from build123d import *

# Parameters (mm, degrees)
CROQUIS18_W                  = 39
CROQUIS18_H                  = 54
SALIENTE_EXTRUIR8_DEPTH      = 40.280661595
SALIENTE_EXTRUIR9_REACH      = 87.298
SALIENTE_EXTRUIR9_END_RADIUS = 16
SALIENTE_EXTRUIR10_DEPTH     = 26.5
CORTAR_EXTRUIR8_START        = -39
CROQUIS22_R                  = 15
CORTAR_EXTRUIR8_DEPTH        = 39
CORTAR_EXTRUIR9_DEPTH        = 84.025081472
CROQUIS24_W                  = 10.8
CROQUIS24_H                  = 54
CORTAR_EXTRUIR10_DEPTH       = 12
CROQUIS25_R                  = 2.25
CORTAR_EXTRUIR11_DEPTH       = 24.2
REDONDEO1_R                  = 2
REDONDEO2_R                  = 2
CROQUIS26_R                  = 2.25
CORTAR_EXTRUIR12_DEPTH       = 30
CROQUIS27_W                  = 15
CROQUIS27_H                  = 15
CORTAR_EXTRUIR13_DEPTH       = 101.562974791


with BuildPart() as part:
    # Croquis18 → Saliente-Extruir8 (new body)
    with BuildSketch(Plane(origin=(0, 0, 0), x_dir=(1, 0, 0), z_dir=(0, 1, 0))):
        with Locations((49.353088131, -3.207737261)):
            Rectangle(CROQUIS18_W, CROQUIS18_H)
    extrude(amount=SALIENTE_EXTRUIR8_DEPTH)

    # Saliente-Extruir9: up to this cylinder (the profile starts outside it)
    saliente_extruir9_end = Plane(origin=(39.1607, 58.280661595, 3.207737261), z_dir=(1, 0, 0)) * Cylinder(SALIENTE_EXTRUIR9_END_RADIUS, 207.596, mode=Mode.PRIVATE)
    # Croquis20 → Saliente-Extruir9 (add, up to the surface)
    with BuildSketch(Plane(origin=(0, 40.280661595, 0), x_dir=(1, 0, 0), z_dir=(0, 1, 0)), mode=Mode.PRIVATE) as saliente_extruir9_sk1:
        Polygon((38.853088131, -11.507737261), (38.853088131, -14.207737261), (60.353088131, -14.207737261), (60.353088131, 7.792262739), (38.853088131, 7.792262739), (38.853088131, 5.092262739), (56.853088131, 5.092262739), (56.853088131, -11.507737261), align=None)
    saliente_extruir9_tool1 = extrude(saliente_extruir9_sk1.sketch, amount=SALIENTE_EXTRUIR9_REACH, mode=Mode.PRIVATE) - saliente_extruir9_end
    add(saliente_extruir9_tool1.solids().sort_by_distance((39.1607, 40.280662, 12.857737))[0])

    # Croquis21 → Saliente-Extruir10 (add)
    with BuildSketch(Plane(origin=(0, 40.280661595, 0), x_dir=(1, 0, 0), z_dir=(0, 1, 0))):
        Polygon((68.853088131, 23.792262739), (29.853088131, 23.792262739), (29.853088131, 7.792262739), (60.353088131, 7.792262739), (60.353088131, -14.207737261), (29.853088131, -14.207737261), (29.853088131, -30.207737261), (68.853088131, -30.207737261), align=None)
    extrude(amount=SALIENTE_EXTRUIR10_DEPTH)

    # Croquis22 → Cortar-Extruir8 (cut)
    with BuildSketch(Plane(origin=(68.853088131, 0, 0), x_dir=(0, 0, -1), z_dir=(1, 0, 0)).offset(CORTAR_EXTRUIR8_START)):
        with Locations((-3.207737261, 58.280661595)):
            Circle(CROQUIS22_R)
    extrude(amount=CORTAR_EXTRUIR8_DEPTH, mode=Mode.SUBTRACT)

    # Croquis23 → Cortar-Extruir9 (cut, through all)
    with BuildSketch(Plane(origin=(68.853088131, 0, 0), x_dir=(0, 0, -1), z_dir=(1, 0, 0))):
        with BuildLine():
            Line((-15.566944355, 66.780661595), (-18.207737261, 66.780661595))
            Line((-18.207737261, 66.780661595), (-18.207737261, 58.280661595))
            ThreePointArc((-18.207737261, 58.280661595), (-17.532333353, 62.731048859), (-15.566944355, 66.780661595))
        make_face()
        with BuildLine():
            ThreePointArc((9.151469833, 66.780661595), (11.116858831, 62.731048859), (11.792262739, 58.280661595))
            Line((11.792262739, 58.280661595), (11.792262739, 66.780661595))
            Line((11.792262739, 66.780661595), (9.151469833, 66.780661595))
        make_face()
    extrude(amount=-CORTAR_EXTRUIR9_DEPTH, mode=Mode.SUBTRACT)

    # Croquis24 → Cortar-Extruir10 (cut)
    with BuildSketch(Plane(origin=(0, 66.780661595, 0), x_dir=(1, 0, 0), z_dir=(0, 1, 0))):
        with Locations((35.253088131, -3.207737261)):
            Rectangle(CROQUIS24_W, CROQUIS24_H)
    extrude(amount=-CORTAR_EXTRUIR10_DEPTH, mode=Mode.SUBTRACT)

    # Croquis25 → Cortar-Extruir11 (cut)
    with BuildSketch(Plane.ZY.offset(-40.653088131)):
        with Locations(Location((20.707737261, 58.280661595, 0), (0, 0, 270))):
            Circle(CROQUIS25_R)
        with Locations(Location((-14.292262739, 58.280661595, 0), (0, 0, 270))):
            Circle(CROQUIS25_R)
    extrude(amount=-CORTAR_EXTRUIR11_DEPTH, mode=Mode.SUBTRACT)

    # Redondeo1
    redondeo1_edges = [part.edges().sort_by_distance(p)[0] for p in [
        (68.853088131, 62.530661595, 18.207737261),
        (68.853088131, 62.530661595, -11.792262739),
        (68.853088131, 33.390330798, -23.792262739),
        (54.753088131, 66.780661595, 30.207737261),
        (29.853088131, 27.390330798, 30.207737261),
        (68.853088131, 33.390330798, 30.207737261),
        (29.853088131, 27.390330798, -23.792262739),
        (29.853088131, 51.200842989, -10.016338076),
        (29.853088131, 54.780661595, -17.585238812),
        (29.853088131, 54.780661595, 24.000713334),
        (40.653088131, 60.780661595, -23.792262739),
        (35.253088131, 54.780661595, -23.792262739),
        (35.253088131, 54.780661595, 30.207737261),
        (40.653088131, 60.780661595, 30.207737261),
        (29.853088131, 40.280661595, 3.207737261),
        (49.353088131, 0, -23.792262739),
        (68.853088131, 0, 3.207737261),
        (68.853088131, 66.780661595, 24.207737261),
        (54.753088131, 66.780661595, -23.792262739),
        (49.353088131, 0, 30.207737261),
        (29.853088131, 0, 3.207737261),
        (29.853088131, 44.181642082, -7.792262739),
        (29.853088131, 44.181642082, 14.207737261),
        (29.853088131, 51.200842989, 16.431812597),
        (68.853088131, 43.280661596, 3.207737261),
        (68.853088131, 66.780661595, -17.792262739),
    ]]
    fillet(redondeo1_edges, radius=REDONDEO1_R)

    # Redondeo2
    # the kernel refuses this fillet: 2 mm, written as the material it takes off along each edge
    with BuildSketch(Plane(origin=(66.853088131, 64.780661595, -13.792262739), x_dir=(0, 1, 0), z_dir=(0, 0, 1))) as redondeo2_piece_1_section:
        Polygon((0, 0), (REDONDEO2_R, 0), (REDONDEO2_R, -REDONDEO2_R), (0, -REDONDEO2_R), align=None)
    redondeo2_piece_1 = extrude(amount=REDONDEO2_R, mode=Mode.PRIVATE)
    redondeo2_piece_1 = redondeo2_piece_1 - Plane(origin=(66.853088131, 64.780661595, -13.792262739), x_dir=(-0.7071067811865475, -0.7071067811865476, 0), z_dir=(0, 0, 1)) * Sphere(REDONDEO2_R, mode=Mode.PRIVATE)
    add(redondeo2_piece_1, mode=Mode.SUBTRACT)
    with BuildSketch(Plane(origin=(66.853088131, 64.780661595, 20.207737261), x_dir=(0, 0, -1), z_dir=(0, 1, 0))) as redondeo2_piece_2_section:
        Polygon((0, 0), (REDONDEO2_R, 0), (REDONDEO2_R, -REDONDEO2_R), (0, -REDONDEO2_R), align=None)
    redondeo2_piece_2 = extrude(amount=REDONDEO2_R, mode=Mode.PRIVATE)
    redondeo2_piece_2 = redondeo2_piece_2 - Plane(origin=(66.853088131, 64.780661595, 20.207737261), x_dir=(-0.7071067811865475, 0, 0.7071067811865475), z_dir=(0, 1, 0)) * Sphere(REDONDEO2_R, mode=Mode.PRIVATE)
    add(redondeo2_piece_2, mode=Mode.SUBTRACT)
    with BuildSketch(Plane(origin=(42.653088131, 64.780661595, -21.792262739), x_dir=(0, 1, 0), z_dir=(-1, 0, 0))) as redondeo2_piece_3_section:
        Polygon((0, 0), (REDONDEO2_R, 0), (REDONDEO2_R, REDONDEO2_R), (0, REDONDEO2_R), align=None)
    redondeo2_piece_3 = extrude(amount=REDONDEO2_R, mode=Mode.PRIVATE)
    redondeo2_piece_3 = redondeo2_piece_3 - Plane(origin=(42.653088131, 64.780661595, -21.792262739), x_dir=(0, -0.7071067811865475, 0.7071067811865475), z_dir=(-1, 0, 0)) * Sphere(REDONDEO2_R, mode=Mode.PRIVATE)
    add(redondeo2_piece_3, mode=Mode.SUBTRACT)
    with BuildSketch(Plane(origin=(42.653088131, 64.780661595, 28.207737261), x_dir=(-1, 0, 0), z_dir=(0, 1, 0))) as redondeo2_piece_4_section:
        Polygon((0, 0), (REDONDEO2_R, 0), (REDONDEO2_R, REDONDEO2_R), (0, REDONDEO2_R), align=None)
    redondeo2_piece_4 = extrude(amount=REDONDEO2_R, mode=Mode.PRIVATE)
    redondeo2_piece_4 = redondeo2_piece_4 - Plane(origin=(42.653088131, 64.780661595, 28.207737261), x_dir=(0.7071067811865475, 0, -0.7071067811865476), z_dir=(0, 1, 0)) * Sphere(REDONDEO2_R, mode=Mode.PRIVATE)
    add(redondeo2_piece_4, mode=Mode.SUBTRACT)
    with BuildSketch(Plane(origin=(66.853088131, 66.780661595, 18.207737261), x_dir=(0, -1.5546675058430992e-10, 1.0), z_dir=(-1, 0, 0)), Plane(origin=(66.853088131, 66.780661595, -11.792262739), x_dir=(0, -1, 0), z_dir=(-1, 0, 0))) as redondeo2_piece_5:
        with BuildLine():
            CenterArc((REDONDEO2_R, -REDONDEO2_R), REDONDEO2_R, 90.000000009, 90)
            Line((REDONDEO2_R * 1.55466750608e-10, -REDONDEO2_R), (0, 0))
            Line((0, 0), (REDONDEO2_R, 0))
        make_face()
    extrude(amount=31.200000001, mode=Mode.SUBTRACT)
    with BuildSketch(Plane(origin=(40.653088131, 66.780661595, -6.792262738), x_dir=(0, -1, 0), z_dir=(0, 0, -1))) as redondeo2_piece_6:
        with BuildLine():
            CenterArc((REDONDEO2_R, -REDONDEO2_R), REDONDEO2_R, 90, 90)
            Line((0, -REDONDEO2_R), (0, 0))
            Line((0, 0), (REDONDEO2_R, 0))
        make_face()
    extrude(amount=15.000000001, mode=Mode.SUBTRACT)
    with BuildSketch(Plane(origin=(40.653088131, 66.780661595, 28.207737261), x_dir=(1.0, -1.5546675058430992e-10, 0), z_dir=(0, 0, -1))) as redondeo2_piece_7:
        with BuildLine():
            CenterArc((REDONDEO2_R, REDONDEO2_R), REDONDEO2_R, 179.999999991, 90)
            Line((REDONDEO2_R * 1.55466750608e-10, REDONDEO2_R), (0, 0))
            Line((0, 0), (REDONDEO2_R, 0))
        make_face()
    extrude(amount=15.000000001, mode=Mode.SUBTRACT)

    # Croquis26 → Cortar-Extruir12 (cut)
    with BuildSketch(Plane.XZ):
        with Locations(Location((39.853088131, 20.207737261, 0), (0, 0, 270))):
            Circle(CROQUIS26_R)
        with Locations(Location((58.853088131, 20.207737261, 0), (0, 0, 270))):
            Circle(CROQUIS26_R)
        with Locations(Location((39.853088131, -13.792262739, 0), (0, 0, 270))):
            Circle(CROQUIS26_R)
        with Locations(Location((58.853088131, -13.792262739, 0), (0, 0, 270))):
            Circle(CROQUIS26_R)
    extrude(amount=-CORTAR_EXTRUIR12_DEPTH, mode=Mode.SUBTRACT)

    # Croquis27 → Cortar-Extruir13 (cut, through all)
    with BuildSketch(Plane.XZ):
        with Locations((49.353088131, 3.207737261)):
            Rectangle(CROQUIS27_W, CROQUIS27_H)
    extrude(amount=-CORTAR_EXTRUIR13_DEPTH, mode=Mode.SUBTRACT)


solid = part.part
Check sheet for the modelled part. Datum: model origin and axes. Units: mm. A direction names the side the tool comes from. Give positions to 0.01 mm unless a question says otherwise; leave off trailing zeros. Loops run counter-clockwise (first coordinate to the right, second up) from the corner with the lowest first, then second, coordinate; pieces in that order, holes last. Notation, with made-up numbers: M -4.75,34 L 30.25,34 A19 ccw 30.25,65 Z; hole C 79.5,-6.75 d11. An arc over 180 degrees is marked long. Answer as a JSON object with one key per item and string values. Group by question number.
Q1. Cross-section at C-C on x = 46. Record the cut outline in (y, z), then the cut area to 3 significant figures.
Q2. Cross-section at D-D on y = 59.5. Record the cut outline in (x, z), then the cut area to 3 significant figures.
Q3. Release check for a two-part mould opening along X. For faces 1 (the cylindrical face through (52.58, 58.57, 22.94)), 2 (the cylindrical face through (68.28, 61.58, -12.39)), 3 (the flat face through (40, 30, -14)) record: released by +X, released by -X, zero draft, split by the parting line, or undercut.
Q4. Access from +Z, -Z, +X, -X, +Y, -Y to the whole of each face (thin tool, end or side, straight path). Record for faces 4 (the flat face through (48, 42, 11.508)), 5 (the flat face through (54, 61, -11.792)), 6 (the flat face through (36, 54.781, -17)), 7 (the flat face through (59, 30, -14)).
Q5. Material ranges on line 1 along Z through (x, y) = (55, 20); line 2 along Z through (x, y) = (35.5, 44.5); line 3 along X through (y, z) = (11, 0), recorded low to high. Write a range as [from, to].
Q6. Cross-section at B-B on z = 26.5. Record the cut outline in (x, y).
Q7. Go/stop test with flat-tipped pins: P1, Ø2, axis at y = 57.5, z = 20, coming from the -X side; P2, Ø6, axis at y = 58.28, z = 20.71, coming from the -X side; P3, Ø5, axis at x = 59.5, z = -13.5, coming from the -Y side; P4, Ø4.5, axis at y = 44, z = 5, coming from the -X side. Record where each tip stops, or that it passes through.
Q8. Cross-section at A-A on y = 34.5. Record the cut outline in (x, z), then the cut area to 3 significant figures.
Evaluation:
{
 "1": {"outline": "M 0,-21.79 A2 ccw 2,-23.79 L 64.78,-23.79 A2 ccw 66.78,-21.79 L 66.78,-13.79 A2 ccw 64.78,-11.79 L 58.28,-11.79 A15 cw 48.08,-7.79 L 46.66,-7.79 A16 cw 44.6,-5.09 L 40.28,-5.09 L 40.28,-4.29 L 0,-4.29 Z; M 0,10.71 L 40.28,10.71 L 40.28,11.51 L 44.6,11.51 A16 cw 46.66,14.21 L 48.08,14.21 A15 cw 58.28,18.21 L 64.78,18.21 A2 ccw 66.78,20.21 L 66.78,28.21 A2 ccw 64.78,30.21 L 2,30.21 A2 ccw 0,28.21 Z; hole C 58.28,-14.29 d4.5; hole C 58.28,20.71 d4.5", "area": "2,290 mm2"},
 "2": {"outline": "M 40.65,-21.79 A2 ccw 42.65,-23.79 L 66.85,-23.79 A2 ccw 68.85,-21.79 L 68.85,-13.79 A2 ccw 66.85,-11.79 L 40.65,-11.79 L 40.65,-12.4 L 64.85,-12.4 L 64.85,-16.18 L 40.65,-16.18 Z; M 40.65,18.21 L 66.85,18.21 A2 ccw 68.85,20.21 L 68.85,28.21 A2 ccw 66.85,30.21 L 42.65,30.21 A2 ccw 40.65,28.21 L 40.65,22.6 L 64.85,22.6 L 64.85,18.82 L 40.65,18.82 Z", "area": "489 mm2"},
 "3": {"face 1": "zero draft", "face 2": "released by +X", "face 3": "undercut"},
 "4": {"face 4": "-X, +Y", "face 5": "+X, -X, +Y", "face 6": "+Z, -Z, -X, +Y", "face 7": "-Y"},
 "5": {"line 1": "z = [-23.79, -4.29], [10.71, 30.21]", "line 2": "z = [-23.79, -7.79], [14.21, 30.21]", "line 3": "x = [29.85, 41.85], [56.85, 68.85]"},
 "6": {"outline": "M 29.85,2 A2 ccw 31.85,0 L 66.85,0 A2 ccw 68.85,2 L 68.85,64.78 A2 ccw 66.85,66.78 L 42.65,66.78 A2 ccw 40.65,64.78 L 40.65,54.78 L 31.85,54.78 A2 ccw 29.85,52.78 Z"},
 "7": {"P1": "stops at x = 64.85", "P2": "stops at x = 40.65", "P3": "stops at y = 0", "P4": "stops at x = 56.85"},
 "8": {"outline": "M 29.85,-21.79 A2 ccw 31.85,-23.79 L 66.85,-23.79 A2 ccw 68.85,-21.79 L 68.85,28.21 A2 ccw 66.85,30.21 L 31.85,30.21 A2 ccw 29.85,28.21 Z; hole M 41.85,-4.29 L 56.85,-4.29 L 56.85,10.71 L 41.85,10.71 Z", "area": "1,880 mm2"}
}
